from build123d import *

# Parameters (mm, degrees)
A_BASE_T42_OUTLINE_R       = 2.2479
A_BASE_T42_OUTLINE_R_2     = 1
A_BASE_T42_DEPTH           = 3
OUTER_BRIM_DEPTH           = 3
SKETCH5_W                  = 15
SKETCH5_H                  = 3
BASE_SUPPORTS_DEPTH        = 3
BASE_SUPPORTS_CHAMFER_SIZE = 3
COVER_START                = -3
SKETCH6_R                  = 1
COVER_DEPTH                = 3
SKETCH9_W                  = 15
SKETCH9_H                  = 6
CUT_EXTRUDE1_DEPTH         = 10
SKETCH11_W                 = 10
SKETCH11_H                 = 10
BOSS_EXTRUDE1_DEPTH        = 4.6
BOSS_EXTRUDE2_DEPTH        = 10.6
FILLET1_R                  = 1
FILLET2_R                  = 5


# Read off the part's stored shape, not the designer's step: a_base_t42
# Some blends are built 0.0001 mm under size
with BuildPart() as part:
    # a_base_t42 outline → a_base_t42 (new body)
    with BuildSketch(Plane(origin=(0, 0, 0), x_dir=(1, 0, 0), z_dir=(0, 1, 0))):
        with BuildLine():
            ThreePointArc((31.5, -42), (52.5, 0), (31.5, 42))
            Line((31.5, 42), (-31.5, 42))
            ThreePointArc((-31.5, 42), (-52.5, 0), (-31.5, -42))
            Line((-31.5, -42), (31.5, -42))
        make_face()
        with Locations((-23, -35)):
            Circle(A_BASE_T42_OUTLINE_R, mode=Mode.SUBTRACT)
        with Locations((23, -35)):
            Circle(A_BASE_T42_OUTLINE_R, mode=Mode.SUBTRACT)
        with Locations((-40.25, 0)):
            Circle(A_BASE_T42_OUTLINE_R_2, mode=Mode.SUBTRACT)
        with Locations((-23, 35)):
            Circle(A_BASE_T42_OUTLINE_R, mode=Mode.SUBTRACT)
        with Locations((40.25, 0)):
            Circle(A_BASE_T42_OUTLINE_R_2, mode=Mode.SUBTRACT)
        with Locations((23, 35)):
            Circle(A_BASE_T42_OUTLINE_R, mode=Mode.SUBTRACT)
    extrude(amount=A_BASE_T42_DEPTH)

    # Sketch1 → Outer Brim (add)
    with BuildSketch(Plane(origin=(0, 3, 0), x_dir=(1, 0, 0), z_dir=(0, 1, 0))):
        with BuildLine():
            Line((-31.5, -42), (31.5, -42))
            ThreePointArc((31.5, -42), (52.5, 0), (31.5, 42))
            Line((31.5, 42), (-31.5, 42))
            ThreePointArc((-31.5, 42), (-52.5, 0), (-31.5, -42))
        make_face()
        with BuildLine():
            Line((30.483602149, 39), (-30.483602149, 39))
            ThreePointArc((-30.483602149, 39), (-49.5, 0), (-30.483602149, -39))
            Line((-30.483602149, -39), (30.483602149, -39))
            ThreePointArc((30.483602149, -39), (49.5, 0), (30.483602149, 39))
        make_face(mode=Mode.SUBTRACT)
    extrude(amount=OUTER_BRIM_DEPTH)

    # Sketch5 → Base Supports (add)
    with BuildSketch(Plane(origin=(0, 3, 0), x_dir=(1, 0, 0), z_dir=(0, 1, 0))):
        with Locations((0, -27)):
            Rectangle(SKETCH5_W, SKETCH5_H)
        with Locations((0, 27)):
            Rectangle(SKETCH5_W, SKETCH5_H)
    extrude(amount=BASE_SUPPORTS_DEPTH)

    # Base Supports Chamfer
    base_supports_chamfer_edges = [part.edges().sort_by_distance(p)[0] for p in [
        (0, 3, 28.5),
        (0, 3, -28.5),
    ]]
    chamfer(base_supports_chamfer_edges, length=BASE_SUPPORTS_CHAMFER_SIZE - 0.0001)  # a hair under: the kernel refuses the full size

    # Sketch6 → Cover (add)
    with BuildSketch(Plane(origin=(0, 3, 0), x_dir=(1, 0, 0), z_dir=(0, 1, 0)).offset(COVER_START)):
        with Locations((-40.25, 0)):
            Circle(SKETCH6_R)
        with Locations((40.25, 0)):
            Circle(SKETCH6_R)
    extrude(amount=COVER_DEPTH)

    # Sketch9 → Cut-Extrude1 (cut)
    with BuildSketch(Plane(origin=(0, 3, 0), x_dir=(1, 0, 0), z_dir=(0, 1, 0))):
        with Locations((0, 28.5)):
            Rectangle(SKETCH9_W, SKETCH9_H)
        with Locations((0, -28.5)):
            Rectangle(SKETCH9_W, SKETCH9_H)
    extrude(amount=CUT_EXTRUDE1_DEPTH, mode=Mode.SUBTRACT)

    # Sketch11 → Boss-Extrude1 (add)
    with BuildSketch(Plane(origin=(5.553919153, 3, -19.484186112), x_dir=(-1, 0, 0), z_dir=(0, 1, 0))):
        with Locations((11.903919153, 39.434186112)):
            Rectangle(SKETCH11_W, SKETCH11_H)
        with Locations((36.303919153, 39.434186112)):
            Rectangle(SKETCH11_W, SKETCH11_H)
        with Locations((36.303919153, 2.534186112)):
            Rectangle(SKETCH11_W, SKETCH11_H)
        with Locations((11.903919153, 2.534186112)):
            Rectangle(SKETCH11_W, SKETCH11_H)
        with Locations((-0.796080847, -0.465813888)):
            Rectangle(SKETCH11_W, SKETCH11_H)
        with Locations((-0.796080847, 36.434186112)):
            Rectangle(SKETCH11_W, SKETCH11_H)
        with Locations((-25.196080847, 36.434186112)):
            Rectangle(SKETCH11_W, SKETCH11_H)
        with Locations((-25.196080847, -0.465813888)):
            Rectangle(SKETCH11_W, SKETCH11_H)
    extrude(amount=BOSS_EXTRUDE1_DEPTH)

    # Sketch13 → Boss-Extrude2 (add)
    with BuildSketch(Plane(origin=(5.553919153, 3, -19.484186112), x_dir=(-1, 0, 0), z_dir=(0, 1, 0))):
        Polygon((2.903919153, 48.434186112), (2.903919153, 45.434186112), (-30.196080847, 45.434186112), (-30.196080847, 41.434186112), (4.203919153, 41.434186112), (4.203919153, 29.434186112), (6.903919153, 29.434186112), (6.903919153, 44.434186112), (16.903919153, 44.434186112), (16.903919153, 48.434186112), align=None)
        Polygon((41.303919153, -2.465813888), (41.303919153, -6.465813888), (8.203919153, -6.465813888), (8.203919153, -9.465813888), (-5.796080847, -9.465813888), (-5.796080847, -5.465813888), (4.203919153, -5.465813888), (4.203919153, 9.534186112), (6.903919153, 9.534186112), (6.903919153, -2.465813888), align=None)
        Polygon((41.303919153, 44.434186112), (41.303919153, 28.434186112), (45.303919153, 28.434186112), (45.303919153, 48.434186112), (31.303919153, 48.434186112), (31.303919153, 44.434186112), align=None)
        Polygon((-34.196080847, -9.465813888), (-34.196080847, 10.534186112), (-30.196080847, 10.534186112), (-30.196080847, -5.465813888), (-20.196080847, -5.465813888), (-20.196080847, -9.465813888), align=None)
    extrude(amount=BOSS_EXTRUDE2_DEPTH)

    # Fillet1
    fillet1_edges = [part.edges().sort_by_distance(p)[0] for p in [
        (11.35, 5.3, 11.95),
        (25.75, 5.3, 11.95),
        (11.35, 5.3, -14.95),
        (25.75, 5.3, -14.95),
        (0, 13.6, 9.95),
        (-25.75, 5.3, 14.95),
        (-11.35, 5.3, 14.95),
        (-11.35, 5.3, -11.95),
        (-25.75, 5.3, -11.95),
        (-35.75, 5.3, 14.95),
        (1.35, 8.3, -9.95),
        (-1.35, 8.3, -9.95),
        (-1.35, 5.3, -11.95),
        (-11.35, 5.3, -21.95),
        (-25.75, 5.3, -21.95),
        (19.2, 13.6, 25.95),
        (39.75, 13.6, -18.95),
        (4.35, 13.6, -28.95),
        (-2.65, 13.6, -27.45),
        (-19.2, 13.6, -25.95),
        (-35.75, 13.6, -23.95),
        (35.75, 13.6, 23.95),
        (39.75, 8.3, -8.95),
        (11.35, 5.3, 21.95),
        (25.75, 5.3, 21.95),
        (35.75, 5.3, -14.95),
        (1.35, 5.3, 11.95),
        (1.35, 5.3, -14.95),
        (-1.35, 5.3, 14.95),
        (-1.35, 8.3, 9.95),
        (1.35, 8.3, 9.95),
        (35.75, 5.3, 11.95),
        (35.75, 8.3, 25.95),
        (2.65, 13.6, 27.45),
        (2.65, 8.3, 25.95),
        (-32.75, 13.6, 28.95),
        (-39.75, 13.6, 18.95),
        (-39.75, 8.3, 8.95),
        (-35.75, 8.3, -25.95),
        (25.75, 8.3, -28.95),
        (11.35, 8.3, -28.95),
        (-11.35, 8.3, 28.95),
        (-25.75, 8.3, 28.95),
    ]]
    fillet(fillet1_edges, radius=FILLET1_R - 0.0001)  # a hair under: the kernel refuses the full size

    # Fillet2
    # the kernel refuses this fillet: 5 mm, written as the material it takes off along each edge
    with BuildSketch(Plane(origin=(-34.75, 13.6, 23.95), x_dir=(-1, 0, 0), z_dir=(0, 0, -1))) as fillet2_piece_1:
        with BuildLine():
            CenterArc((4.0001, -0.9999), 0.9999, 0, 90)
            Line((5, -0.9999), (5, 0))
            Line((5, 0), (4.0001, 0))
        make_face()
    revolve(axis=Axis((-34.75, 13.6, 23.95), (0, 1, 0)), revolution_arc=90, mode=Mode.SUBTRACT)
    with BuildSketch(Plane(origin=(-39.75, 3, 28.95), x_dir=(0, 0, -1), z_dir=(0, 1, 0))) as fillet2_piece_2:
        with BuildLine():
            CenterArc((FILLET2_R, -FILLET2_R), FILLET2_R, 90, 90)
            Line((0, -FILLET2_R), (0, 0))
            Line((0, 0), (FILLET2_R, 0))
        make_face()
    extrude(amount=10.6, mode=Mode.SUBTRACT)


solid = part.part
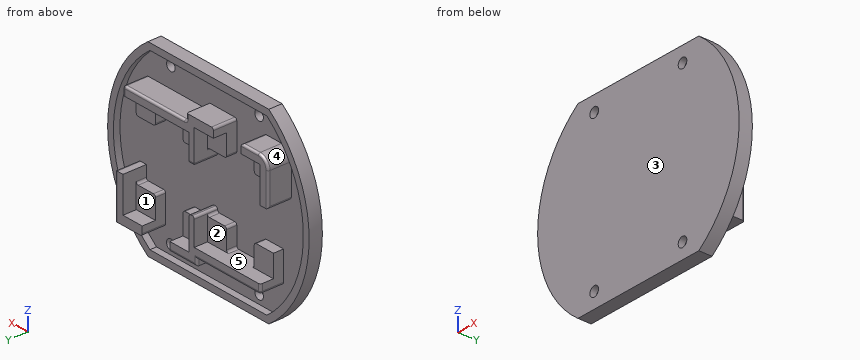
CAD build for the part. Positions are in the model's coordinates, mm. Face numbers are marked on the shaded views. A direction names the side the tool comes from. Coordinates: 2 decimals unless noted, no trailing zeros. Write each loop counter-clockwise with the first axis right and the second up, starting at its lowest first coordinate (ties: lowest second). Pieces come first, ordered by that corner, then holes. Notation, with made-up numbers: M -17,37.5 L -8,37.5 A30 ccw -8,75.5 Z; hole C -27.75,13.25 d8. An arc over 180 degrees is marked long. Answer as a JSON object with one key per item and string values. Group by question number.
1) Saw through at B-B (z = -35). Write the cut outline in (x, y), plus the area to 3 significant figures.
2) Mould opens along X. For the marked faces 3, 4 and 5 say: +X half, -X half, draft (parallel to the pull), parting line (faces both ways), or undercut.
3) Wall check: line 1 (Z direction, x = 23, y = 1.35); line 2 (Z direction, x = -13, y = 5.75); line 3 (Z direction, x = -9.5, y = 9). Give the ranges that are in metal, low to high. Write a range as from..to.
4) Saw through at C-C (y = 11.5). Give the number of separate pieces and of enclosed holes in the cut face, plus the area to 3 significant figures.
5) Pin check, flat tips, straight feed: pin 1 Ø5 at (y, z) = (9.5, -17) entering from -X; pin 2 Ø3 at (y, z) = (9.5, 22.5) entering from +X; pin 3 Ø10 at (x, z) = (-35.5, -8) entering from +Y. Stop position of each tip, or through.
6) Tool access for the marked faces 1 and 2: list every direction of +Z, -Z, +X, -X, +Y, -Y with a clear straight run to the whole face (end or side of a thin tool).
7) Saw through at D-D (x = 45.5). Write the cut outline in (y, z).
8) Saw through at A-A (x = 23). Write the cut outline in (y, z).
Values follow:
{
 "1": {"outline": "M -39.13,0 L -25.25,0 L -25.25,3 L -35,3 L -35,6 L -39.13,6 Z; M -20.75,0 L 20.75,0 L 20.75,3 L -20.75,3 Z; M 25.25,0 L 39.13,0 L 39.13,6 L 35,6 L 35,3 L 25.25,3 Z", "area": "233 mm2"},
 "2": {"face 3": "draft", "face 4": "undercut", "face 5": "undercut"},
 "3": {"line 1": "z = -42..-37.25, -32.75..32.75, 37.25..42", "line 2": "z = -42..-39, -25.95..-21.95, 39..42", "line 3": "z = -25.95..-21.95, 24.95..28.95"},
 "4": {"separate pieces": "4", "enclosed holes": "0", "area": "698 mm2"},
 "5": {"pin 1": "stops at x = -35.75", "pin 2": "stops at x = 35.75", "pin 3": "stops at y = 7.6"},
 "6": {"face 1": "+Y", "face 2": "-X, +Y"},
 "7": {"outline": "M 0,-26.19 L 6,-26.19 L 6,-19.49 L 3,-19.49 L 3,19.49 L 6,19.49 L 6,26.19 L 0,26.19 Z"},
 "8": {"outline": "M 0,-42 L 6,-42 L 6,-39 L 3,-39 L 3,-37.25 L 0,-37.25 Z; M 0,-32.75 L 3,-32.75 L 3,21.95 L 13.6,21.95 L 13.6,24.95 A1 ccw 12.6,25.95 L 3,25.95 L 3,32.75 L 0,32.75 Z; M 0,37.25 L 3,37.25 L 3,39 L 6,39 L 6,42 L 0,42 Z"}
}
